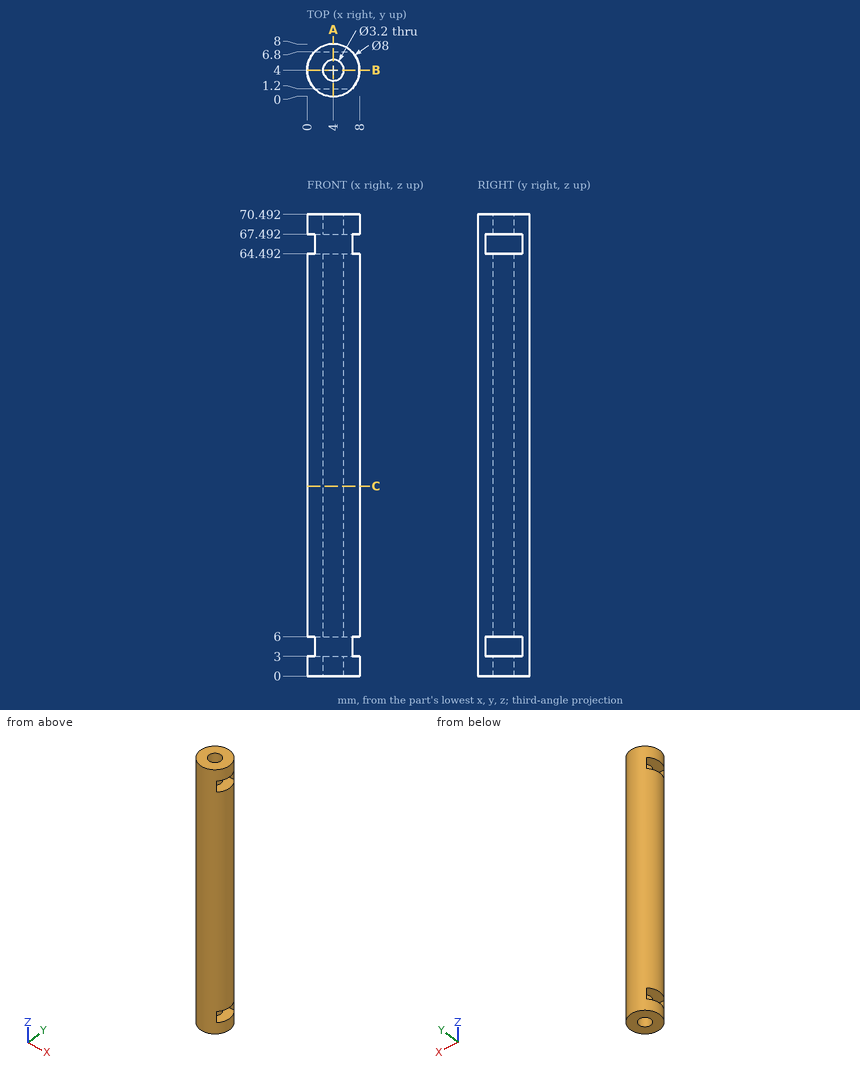
Part print with two shaded views. Sizes in mm from the minimum x, y, z corner. Coordinates: 2 decimals unless noted, no trailing zeros. Write each loop counter-clockwise with the first axis right and the second up, starting at its lowest first coordinate (ties: lowest second). Pieces come first, ordered by that corner, then holes.
(1) Cut at C-C on z = 29. List the corners of the cut face in (x, y).
(2) Cut at B-B on y = 4. List the corners of the cut face in (x, z).
(3) Drill centre lines: line 1 (Z direction, x = 1.75, y = 1.75); line 2 (X direction, y = 4, z = 69); line 3 (Y direction, x = 4.25, z = 49.5). Where is each one in solid material? Low to high.
(4) Cut at A-A on x = 4. List the corners of the cut face in (y, z), and give its area (3 significant figures).
(5) Pin check, flat tips, straight feed: pin 1 Ø3.5 at (x, z) = (5, 5) entering from -Y; pin 2 Ø1.9 at (x, y) = (4, 4) entering from -Z; pin 3 Ø1 at (x, z) = (3, 27.5) entering from +Y; pin 4 Ø1.5 at (x, z) = (6.5, 32.5) entering from +Y. Stop position of each tip, or through.
Working result:
1. outline: circle Ø8 at (4, 4); hole circle Ø3.2 at (4, 4)
2. outline: (0, 0) - (2.4, 0) - (2.4, 3) - (0, 3) - close; (0, 6) - (2.4, 6) - (2.4, 64.49) - (0, 64.49) - close; (0, 67.49) - (2.4, 67.49) - (2.4, 70.49) - (0, 70.49) - close; (5.6, 0) - (8, 0) - (8, 3) - (5.6, 3) - close; (5.6, 6) - (8, 6) - (8, 64.49) - (5.6, 64.49) - close; (5.6, 67.49) - (8, 67.49) - (8, 70.49) - (5.6, 70.49) - close
3. line 1: z = 0 to 3, 6 to 64.49, 67.49 to 70.49
3. line 2: x = 0 to 2.4, 5.6 to 8
3. line 3: y = 0.01 to 2.42, 5.58 to 7.99
4. outline: (0, 0) - (2.4, 0) - (2.4, 3) - (1.2, 3) - (1.2, 6) - (2.4, 6) - (2.4, 64.49) - (1.2, 64.49) - (1.2, 67.49) - (2.4, 67.49) - (2.4, 70.49) - (0, 70.49) - close; (5.6, 0) - (8, 0) - (8, 70.49) - (5.6, 70.49) - (5.6, 67.49) - (6.8, 67.49) - (6.8, 64.49) - (5.6, 64.49) - (5.6, 6) - (6.8, 6) - (6.8, 3) - (5.6, 3) - close
4. area: 324 mm2
5. pin 1: stops at y = 0
5. pin 2: passes through
5. pin 3: stops at y = 7.97
5. pin 4: stops at y = 7.6
